Autodesk Inventor part; units mm, degrees
ref_plane "YZ Plane" through (0, 0, 0) normal (1, 0, 0) x (0, 1, 0)
ref_plane "XZ Plane" through (0, 0, 0) normal (0, 1, 0) x (-1, 0, 0)
ref_plane "XY Plane" through (0, 0, 0) normal (0, 0, 1) x (1, 0, 0)
sketch "Sketch1" plane through (0, 0, 0) normal (0, 1, 0) x (-1, 0, 0)
  circle A0 centre (0, 0) radius 13.5
  circle A1 centre (0, 0) radius 12.5
  dimension "d0" = 27
  dimension "d6" = 25
extrude "Extrusion1" add sketch "Sketch1" along normal blind 160 contours A0 | A1
sketch "Sketch2" plane through (0, 160, 0) normal (0, 1, 0) x (1, 0, 0)
  circle A0 centre (0, 0) radius 13.5
  circle A1 centre (0, 0) radius 12.5
  dimension "d3" = 25
extrude "Extrusion2" cut sketch "Sketch2" against normal blind 65
extrude "Extrusion3" cut sketch "Sketch1" along normal blind 30
fillet "Fillet1" radius 5 1 edges at (-12.5, 160, 0)
thread "Thread1"
thread "Thread2"
properties part number "Stud" material "Steel, High Strength, Low Alloy"
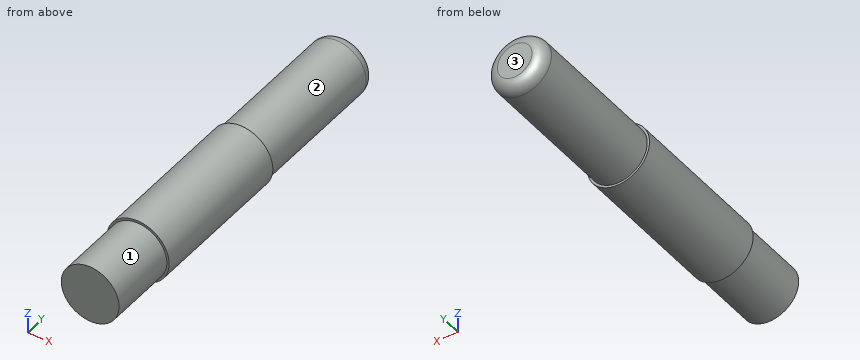
The listing builds one solid part. Answer for the finished solid, in the listing's coordinates (mm). Face numbers are marked on the shaded views. A direction names the side the tool comes from. Give positions to 0.01 mm unless a question says otherwise; leave off trailing zeros. Order: outer loops, then holes, each group sorted by start corner. A loop starts at its lowest first (then second) coordinate and runs counter-clockwise, first axis right, second up.
Item 1: The part is cut by section D-D, the plane y = 130. Give the vertices of the cut face in (x, z), and give its area (3 significant figures).
From the geometry:
outline: circle Ø25 at (0, 0)
area: 491 mm2
Item 2: The part is cut by section B-B, the plane x = 0. Give the vertices of the cut face in (y, z).
From the geometry:
outline: (0, -12.5) - (30, -12.5) - (30, -13.5) - (95, -13.5) - (95, -12.5) - (155, -12.5) arc R5 ccw to (160, -7.5) - (160, 7.5) arc R5 ccw to (155, 12.5) - (95, 12.5) - (95, 13.5) - (30, 13.5) - (30, 12.5) - (0, 12.5) - close
Item 3: The part is cut by section C-C, the plane y = 76. Give the vertices of the cut face in (x, z), and give its area (3 significant figures).
From the geometry:
outline: circle Ø27 at (0, 0)
area: 573 mm2
Item 4: The part is cut by section A-A, the plane z = 0. Give the vertices of the cut face in (x, y), and give its area (3 significant figures).
From the geometry:
outline: (-13.5, 30) - (-12.5, 30) - (-12.5, 0) - (12.5, 0) - (12.5, 30) - (13.5, 30) - (13.5, 95) - (12.5, 95) - (12.5, 155) arc R5 ccw to (7.5, 160) - (-7.5, 160) arc R5 ccw to (-12.5, 155) - (-12.5, 95) - (-13.5, 95) - close
area: 4,120 mm2
Item 5: Which of the six approach directions +Z, -Z, +X, -X, +Y, -Y give full straight-line access (tool end or side, diameter ignored) to the marked faces 1, 2 and 3?
From the geometry:
face 1: -Y
face 2: +Y
face 3: +Z, -Z, +X, -X, +Y
Item 6: Given pin 1 Ø6 at (x, y) = (4.5, 22) entering from +Z; pin 2 Ø12 at (y, z) = (30.5, 10) entering from -X; pin 3 Ø10 at (y, z) = (55, 5.5) entering from +X, each flat-ended and moving along its own axis, determine where each tip first touches the part or whether it passes through.
From the geometry:
pin 1: stops at z = 12.41
pin 2: stops at x = -12.89
pin 3: stops at x = 13.49
Item 7: Find the intervals of material crossed by probe 1 along X at (y, z) = (132, 0); probe 2 along Z at (x, y) = (0.5, 125); probe 3 along Y at (x, z) = (-11.5, -5.25), in increasing order.
From the geometry:
probe 1: x = -12.5 to 12.5
probe 2: z = -12.49 to 12.49
probe 3: y = 30 to 95
